Can you work these out from the model? Positions are in its coordinate system, mm. A direction names the side the tool comes from. Give positions to 0.01 mm unless a question says otherwise; leave off trailing zeros. Write each loop counter-clockwise with the first axis right and the second up, starting at its lowest first coordinate (ties: lowest second). Pieces come first, ordered by that corner, then holes.
1. If I drill on probe 1 along Z at (x, y) = (200, -12.5); probe 2 along Z at (x, y) = (200, -4.35); probe 3 along Y at (x, z) = (121, 237.5), over which ranges is the centre line in solid material (lowest first)?
2. On a 3-axis mill with a long thin cutter (end or side, diameter ignored), from which of +Z, -Z, +X, -X, +Y, -Y can I reach the whole of each face in a straight line? I mean faces 1 (the cylindrical face through (284.94, -12.409, 502.226)), 2 (the flat face through (400, -9, 308)). Say none if no direction works.
3. Thinking about a two-plate mould opening in Z: for faces 3 (the flat face through (197, -19, 178)), 4 (the flat face through (197, -9, 0)), 5 (the flat face through (70.5, -6, 428.3)), which applies, pulls with the +Z half, pulls with the -Z half, needs draft (parallel to the pull), parting line crosses it, or undercut?
4. Suppose I cut it at A-A (x = 200). Please give me the cut outline in (y, z), and give its area (3 significant figures).
5. Suppose I cut it at B-B (z = 369). Please give me the cut outline in (x, y), and give its area (3 significant figures).
6. Suppose I cut it at C-C (y = -10.5). Please give me the cut outline in (x, z), and give its area (3 significant figures).
```python
from build123d import *

# Parameters (mm, degrees)
F0_W     = 400
F0_H     = 624
F0_R     = 158
F1_DEPTH = 19
F0_R_2   = 142
F2_DEPTH = 6


with BuildPart() as f1:
    # F0 (on Front) → F1 (new body)
    with BuildSketch(Plane.XZ):
        with Locations((200, 312)):
            Rectangle(F0_W, F0_H)
        with Locations((200, 369)):
            Circle(F0_R, mode=Mode.SUBTRACT)
    extrude(amount=F1_DEPTH)

    # F0 (on Front) → F2 (join)
    with BuildSketch(Plane.XZ):
        with Locations((200, 369)):
            Circle(F0_R)
        with Locations((200, 369)):
            Circle(F0_R_2, mode=Mode.SUBTRACT)
    extrude(amount=F2_DEPTH)


solid = f1.part
```
Checks:
1. probe 1: z = 0 to 211, 527 to 624
1. probe 2: z = 0 to 227, 511 to 624
1. probe 3: y = -6 to 0
2. face 1: -Y
2. face 2: +Z, -Z, +X, +Y, -Y
3. face 3: needs draft
3. face 4: pulls with the -Z half
3. face 5: undercut
4. outline: (-19, 0) - (0, 0) - (0, 227) - (-6, 227) - (-6, 211) - (-19, 211) - close; (-19, 527) - (-6, 527) - (-6, 511) - (0, 511) - (0, 624) - (-19, 624) - close
4. area: 6,040 mm2
5. outline: (0, -19) - (42, -19) - (42, -6) - (58, -6) - (58, 0) - (0, 0) - close; (342, -6) - (358, -6) - (358, -19) - (400, -19) - (400, 0) - (342, 0) - close
5. area: 1,790 mm2
6. outline: (0, 0) - (400, 0) - (400, 624) - (0, 624) - close; hole circle Ø316 at (200, 369)
6. area: 171,000 mm2
